The listing builds one solid part. Answer for the finished solid, in the listing's coordinates (mm). Face numbers are marked on the shaded views. Round coordinates to 2 decimals unless told otherwise and drop trailing zeros. Loops run counter-clockwise (first coordinate to the right, second up) from the corner with the lowest first, then second, coordinate; pieces in that order, holes last. Notation, with made-up numbers: (59, 77) - (65, 77) arc R24 cw to (65, 103) - close; hole circle Ø2 at (-37.75, 51). An arc over 180 degrees is marked (long way). Write item = value, one per line. Start each with the question number.
1) Section A-A, the plane x = 0 is taken. Determine the outline of the cut face in (y, z).
2) Section B-B, the plane z = -7.25 is taken. Determine the outline of the cut face in (x, y), and give its area (3 significant figures).
3) Given pin 1 Ø5 at (x, y) = (9.5, 44) entering from +Z; pin 2 Ø6.5 at (x, y) = (-12.7, 79.7) entering from +Z; pin 3 Ø2.5 at (x, y) = (-14.5, 46.5) entering from +Z, each flat-ended and moving along its own axis, determine where each tip first touches the part or whether it passes through.
4) Straight lines are drawn through the part: line 1 along X through (y, z) = (79.7, -7.35); line 2 along Y through (x, z) = (12.7, -7.9); line 3 along Y through (x, z) = (11, -7.5). For each, find the intervals that lie inside material, in ascending order.
5) For a pull along Z with two mould halves and no side action, classify the marked faces 1, 2, 3 and 4 as released by +Z, released by -Z, zero draft, split by the parting line, or undercut.
6) Section C-C, the plane y = 3.5 is taken. Give the number of separate pieces and of enclosed holes in the cut face, and give its area (3 significant figures).
from build123d import *

# Parameters (mm, degrees)
SKETCH2_R               = 6.34
SKETCH2_R_2             = 3.84
BOSS_EXTRUDE1_DEPTH     = 83.2
FILLET1_R               = 7.68
CUT_EXTRUDE1_DEPTH      = 89.8622666
CUT_EXTRUDE1_DEPTH_BACK = 89.8622666
SKETCH3_R               = 2


with BuildPart() as part:
    # Sketch2 → Boss-Extrude1 (new body)
    # profile 1 of 2: a face of its own
    with BuildSketch(Plane(origin=(0, 0, 0), x_dir=(1, 0, 0), z_dir=(0, 1, 0))):
        with BuildLine():
            Line((16.2, 10.34), (-16.2, 10.34))
            Line((-16.2, 10.34), (-16.2, 6.34))
            Line((-16.2, 6.34), (-6.34, 6.34))
            Line((-6.34, 6.34), (-6.34, 0))
            ThreePointArc((-6.34, 0), (0, 6.34), (6.34, 0))
            Line((6.34, 0), (6.34, 6.34))
            Line((6.34, 6.34), (16.2, 6.34))
            Line((16.2, 6.34), (16.2, 10.34))
        make_face()
    # profile 2 of 2: a face of its own
    with BuildSketch(Plane(origin=(0, 0, 0), x_dir=(1, 0, 0), z_dir=(0, 1, 0))):
        Circle(SKETCH2_R)
        with Locations(Location((0, 0, 0), (0, 0, 270))):
            Circle(SKETCH2_R_2, mode=Mode.SUBTRACT)
    extrude(amount=BOSS_EXTRUDE1_DEPTH)

    # Fillet1
    fillet1_edges = [part.edges().sort_by_distance(p)[0] for p in [
        (-6.34, 41.6, -6.34),
        (6.34, 41.6, -6.34),
    ]]
    fillet(fillet1_edges, radius=FILLET1_R)

    # Sketch3 → Cut-Extrude1 (cut, two sides: drawn at the far end of the back side and taken through both)
    with BuildSketch(Plane(origin=(0, 0, -20.34), x_dir=(-1, 0, 0), z_dir=(0, 0, -1)).offset(-CUT_EXTRUDE1_DEPTH_BACK)):
        with Locations((12.7, 79.7)):
            Circle(SKETCH3_R)
        with Locations((12.7, 3.5)):
            Circle(SKETCH3_R)
        with Locations((-12.7, 3.5)):
            Circle(SKETCH3_R)
        with Locations((-12.7, 79.7)):
            Circle(SKETCH3_R)
    extrude(amount=CUT_EXTRUDE1_DEPTH + CUT_EXTRUDE1_DEPTH_BACK, mode=Mode.SUBTRACT)


solid = part.part
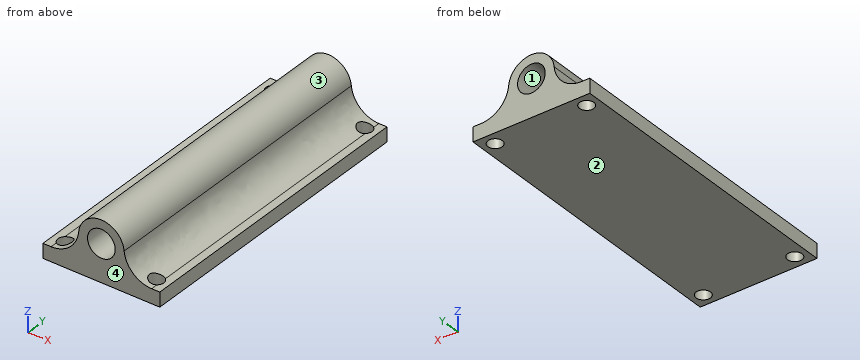
Geometry check:
q1.outline = (0, -10.34) - (83.2, -10.34) - (83.2, -3.84) - (0, -3.84) - close; (0, 3.84) - (83.2, 3.84) - (83.2, 6.34) - (0, 6.34) - close
q2.outline = (-16.2, 0) - (16.2, 0) - (16.2, 83.2) - (-16.2, 83.2) - close; hole circle Ø4 at (-12.7, 3.5); hole circle Ø4 at (-12.7, 79.7); hole circle Ø4 at (12.7, 3.5); hole circle Ø4 at (12.7, 79.7)
q2.area = 2,650 mm2
q3.pin_1 = -1.92
q3.pin_2 = -4.88
q3.pin_3 = -6.31
q4.line_1 = -16.2 to -14.7, -10.7 to 10.7, 14.7 to 16.2
q4.line_2 = 0 to 1.5, 5.5 to 77.7, 81.7 to 83.2
q4.line_3 = 0 to 2.45, 4.55 to 78.65, 80.75 to 83.2
q5.face_1 = undercut
q5.face_2 = released by -Z
q5.face_3 = released by +Z
q5.face_4 = zero draft
q6.separate_pieces = 3
q6.enclosed_holes = 1
q6.area = 218 mm2
